Geometry: final body of the model. Coordinates: model frame, mm. A direction names the side the tool comes from. Round coordinates to 2 decimals unless told otherwise and drop trailing zeros. Loops run counter-clockwise (first coordinate to the right, second up) from the corner with the lowest first, then second, coordinate; pieces in that order, holes last. Notation, with made-up numbers: (-39, 30) - (-32, 30) arc R29 cw to (-32, 64) - close; hole circle Ø4 at (79, 30). An arc over 180 degrees is marked (long way). Return JSON: item names as keys, results as strings. Group by question number.
1. Section D-D on z = -843. Return loops of the section in (x, y).
2. Set-up query: faces 1 (the face through (-21.984, -499.516, 592.098)), 2 (the face through (-206, -94, -1350.9)). Return all of +Z, -Z, +X, -X, +Y, -Y with unobstructed straight access to the full face (end or side cutting, diameter ignored); none if empty.
3. Section A-A on x = 0. Return loops of the section in (y, z), and give its area (3 significant figures).
4. Draft query along Z for faces 3 (the face through (130.56, -170.27, 258.73)), 4 (the face through (-7, 7, 686.4)), 5 (the face through (-449.565, 19.786, -1357.339)). Return one class per face: +Z half, -Z half, draft (parallel to the pull), parting line (faces both ways), or undercut.
5. Section C-C on z = 74. Return loops of the section in (x, y), and give its area (3 significant figures).
6. First-contact query: pin 1 Ø12 at (y, z) = (-130.5, -279) entering from +X; pin 2 Ø12 at (y, z) = (-4, -652) entering from -X; pin 3 Ø3 at (x, z) = (15, 266) entering from +Y. Flat tips, straight axial feed; report the tip coordinate or a pass-through.
7. Material intervals for probe 1 along Z at (x, y) = (-158.5, 110); probe 2 along Z at (x, y) = (-179, 223); probe 3 along X at (y, z) = (-92.5, -1103.5), sorted ascending.
from build123d import *

# Parameters (mm, degrees)
SKETCH1_R                = 50.8
BOSS_EXTRUDE1_DEPTH      = 686.4
BOSS_EXTRUDE1_DEPTH_BACK = 1363.6
SKETCH2_R                = 450
BOSS_EXTRUDE2_DEPTH      = 12.7
SKETCH3_R                = 222.25
BOSS_EXTRUDE3_DEPTH      = 1200


with BuildPart() as part:
    # Sketch1 → Boss-Extrude1 (new body, two sides)
    with BuildSketch(Plane.XY) as boss_extrude1_sk:
        Circle(SKETCH1_R)
    extrude(amount=BOSS_EXTRUDE1_DEPTH)
    extrude(boss_extrude1_sk.sketch, amount=-BOSS_EXTRUDE1_DEPTH_BACK)

    # Sketch2 → Boss-Extrude2 (add)
    with BuildSketch(Plane.XY.offset(-1363.6)):
        Circle(SKETCH2_R)
    extrude(amount=BOSS_EXTRUDE2_DEPTH)

    # Sketch3 → Boss-Extrude3 (add)
    with BuildSketch(Plane.XY.offset(-1350.9)):
        Circle(SKETCH3_R)
    extrude(amount=BOSS_EXTRUDE3_DEPTH)

    # Sketch5 → Revolve1 (revolve)
    with BuildSketch(Plane(origin=(0, 0, 0), x_dir=(0, 0, -1), z_dir=(1, 0, 0))):
        Polygon((-686.4, 0), (-686.4, 500), (-500.4, 500), (-246.4, 200), (-246.4, 0), align=None)
    revolve(axis=Axis((0, 0, 246.4), (0, 0, 1)))


solid = part.part
Taken from the geometry:
{
 "1": {"outline": "circle Ø444.5 at (0, 0)"},
 "2": {"face 1": "+Z, -Z", "face 2": "none"},
 "3": {"outline": "(-500, 500.4) - (-200, 246.4) - (-50.8, 246.4) - (-50.8, -150.9) - (-222.25, -150.9) - (-222.25, -1350.9) - (-450, -1350.9) - (-450, -1363.6) - (450, -1363.6) - (450, -1350.9) - (222.25, -1350.9) - (222.25, -150.9) - (50.8, -150.9) - (50.8, 246.4) - (200, 246.4) - (500, 500.4) - (500, 686.4) - (-500, 686.4) - close", "area": "949,000 mm2"},
 "4": {"face 3": "undercut", "face 4": "+Z half", "face 5": "draft"},
 "5": {"outline": "circle Ø101.6 at (0, 0)", "area": "8,110 mm2"},
 "6": {"pin 1": "x = 184.11", "pin 2": "x = -222.25", "pin 3": "y = 224.42"},
 "7": {"probe 1": "-1363.6 to -150.9, 246.4 to 686.4", "probe 2": "-1363.6 to -1350.9, 319.17 to 686.4", "probe 3": "-202.09 to 202.09"}
}
